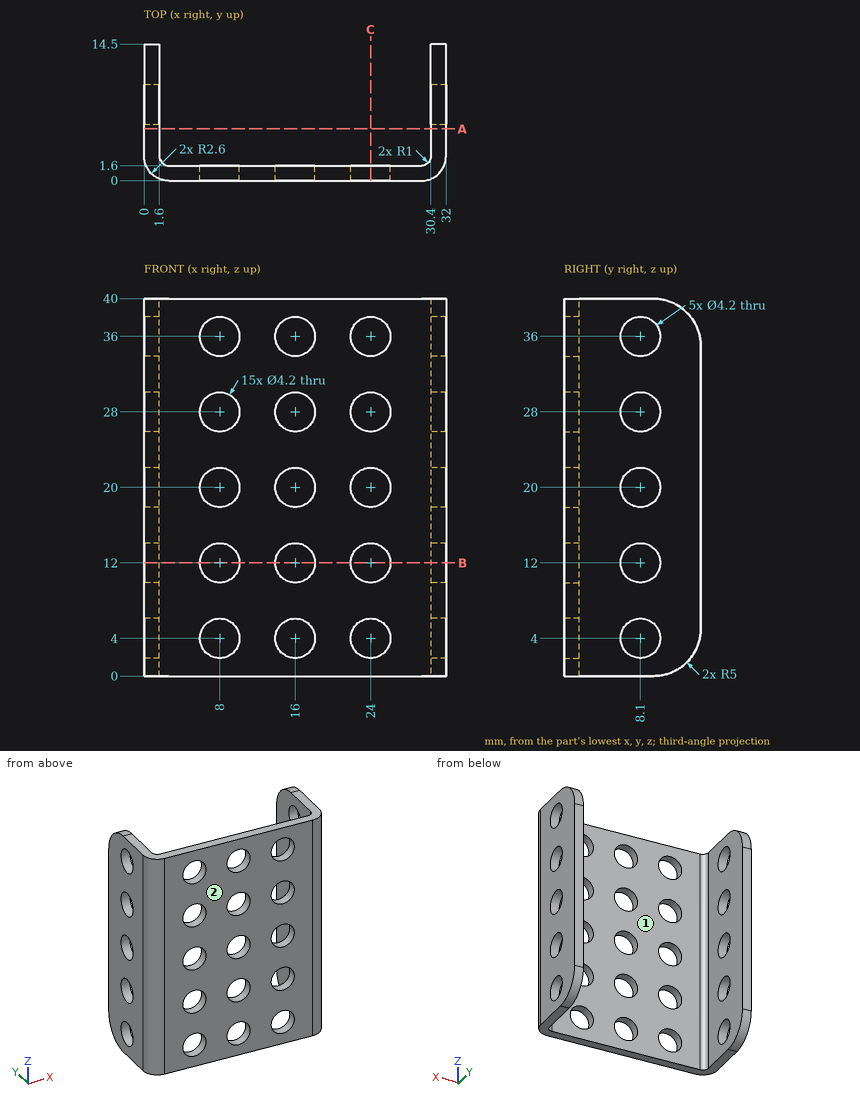
Geometry: see drawing. Coordinates: mm, zero at the bounding-box minimum. A direction names the side the tool comes from. Give positions to 0.01 mm unless a question says otherwise; leave off trailing zeros. Order: outer loops, then holes, each group sorted by start corner. A loop starts at its lowest first (then second) coordinate and runs counter-clockwise, first axis right, second up.
1. Set-up query: the marked faces 1 and 2. Return all of +Z, -Z, +X, -X, +Y, -Y with unobstructed straight access to the full face (end or side cutting, diameter ignored); none if empty.
Computed:
face 1: +Z, -Z, +Y
face 2: +Z, -Z, +X, -X, -Y
2. Cut plane B-B (z = 12). State how many separate pieces and enclosed holes the cut face has, and give its area (3 significant figures).
Computed:
separate pieces: 6
enclosed holes: 0
area: 56.4 mm2
3. Cut plane C-C (x = 24). Return loops of the section in (y, z), and give its area (3 significant figures).
Computed:
outline: (0, 0) - (1.6, 0) - (1.6, 1.9) - (0, 1.9) - close; (0, 6.1) - (1.6, 6.1) - (1.6, 9.9) - (0, 9.9) - close; (0, 14.1) - (1.6, 14.1) - (1.6, 17.9) - (0, 17.9) - close; (0, 22.1) - (1.6, 22.1) - (1.6, 25.9) - (0, 25.9) - close; (0, 30.1) - (1.6, 30.1) - (1.6, 33.9) - (0, 33.9) - close; (0, 38.1) - (1.6, 38.1) - (1.6, 40) - (0, 40) - close
area: 30.4 mm2
4. Cut plane A-A (y = 5.5). Return loops of the section in (x, z), and give its area (3 significant figures).
Computed:
outline: (0, 0) - (1.6, 0) - (1.6, 40) - (0, 40) - close; (30.4, 0) - (32, 0) - (32, 40) - (30.4, 40) - close
area: 128 mm2
5. Line query: probe 1 along Z at (x, y) = (0.6, 8.1); probe 2 along X at (y, z) = (11.75, 10.5); probe 3 along X at (y, z) = (0.9, 12). Output: solid intervals per line, ascending.
Computed:
probe 1: z = 0 to 1.9, 6.1 to 9.9, 14.1 to 17.9, 22.1 to 25.9, 30.1 to 33.9, 38.1 to 40
probe 2: x = 0 to 1.6, 30.4 to 32
probe 3: x = 0.63 to 5.9, 10.1 to 13.9, 18.1 to 21.9, 26.1 to 31.37
6. Pin query (flat end, axial travel): pin 1 Ø5.5 at (x, z) = (8, 4) entering from +Y; pin 2 Ø6.5 at (y, z) = (8.1, 12) entering from +X. Return the tip coordinate at first contact, or that it passes through.
Computed:
pin 1: stops at y = 1.6
pin 2: stops at x = 32
